from build123d import *

# Parameters (mm, degrees)
ESQUISSE1_R             = 0.65
BOSS_EXTRU_1_DEPTH      = 1
BOSS_EXTRU_2_DEPTH      = 0.6
ESQUISSE4_R             = 0.7
BOSS_EXTRU_3_DEPTH      = 1.8
CHANFREIN1_SIZE         = 0.05
CHANFREIN2_SIZE         = 0.05
ESQUISSE5_R             = 0.575
ENL_V_MAT_EXTRU_1_DEPTH = 2.4
ESQUISSE6_R             = 0.55
ENL_V_MAT_EXTRU_2_DEPTH = 2.4
CHANFREIN3_SIZE         = 0.05
CHANFREIN4_SIZE         = 0.05
CHANFREIN5_SIZE         = 0.01
ESQUISSE7_R             = 0.075
BOSS_EXTRU_4_DEPTH      = 1.5
ECHELLE1_SCALE          = 10


with BuildPart() as part:
    # Esquisse1 → Boss.-Extru.1 (new body)
    with BuildSketch(Plane(origin=(0, 0, 0), x_dir=(0, 0, -1), z_dir=(1, 0, 0))):
        Circle(ESQUISSE1_R)
    extrude(amount=BOSS_EXTRU_1_DEPTH)

    # Esquisse2 → Révolution1 (revolve)
    with BuildSketch(Plane.XY):
        with BuildLine():
            Line((0, 0.65), (0.15, 0.65))
            ThreePointArc((0.15, 0.65), (0.075, 0.725), (0, 0.65))
        make_face()
    revolve(axis=Axis((1, 0, 0), (-1, 0, 0)))

    # Esquisse3 → Boss.-Extru.2 (add)
    with BuildSketch(Plane.ZY):
        Polygon((0.713221279, -0.587067918), (0.86502637, 0.324133787), (0.151805091, 0.911201705), (-0.713221279, 0.587067918), (-0.86502637, -0.324133787), (-0.151805091, -0.911201705), align=None)
    extrude(amount=BOSS_EXTRU_2_DEPTH)

    # Esquisse4 → Boss.-Extru.3 (add)
    with BuildSketch(Plane.ZY.offset(0.6)):
        Circle(ESQUISSE4_R)
    extrude(amount=BOSS_EXTRU_3_DEPTH)

    # Chanfrein1
    chanfrein1_edges = [part.edges().sort_by_distance(p)[0] for p in [
        (-0.6, -0.749134812, 0.280708094),
        (-0.6, -0.131467065, 0.789123825),
        (-0.6, 0.617667746, 0.508415731),
        (-0.6, 0.749134812, -0.280708094),
        (-0.6, 0.131467065, -0.789123825),
        (-0.6, -0.617667746, -0.508415731),
    ]]
    chamfer(chanfrein1_edges, length=CHANFREIN1_SIZE)

    # Chanfrein2
    chanfrein2_edges = [part.edges().sort_by_distance(p)[0] for p in [
        (0, 0.749134812, -0.280708094),
        (0, 0.131467065, -0.789123825),
        (0, -0.617667746, -0.508415731),
        (0, -0.749134812, 0.280708094),
        (0, -0.131467065, 0.789123825),
        (0, 0.617667746, 0.508415731),
    ]]
    chamfer(chanfrein2_edges, length=CHANFREIN2_SIZE)

    # Esquisse5 → Enlèv. mat.-Extru.1 (cut)
    with BuildSketch(Plane.ZY.offset(2.4)):
        Circle(ESQUISSE5_R)
    extrude(amount=-ENL_V_MAT_EXTRU_1_DEPTH, mode=Mode.SUBTRACT)

    # Esquisse6 → Enlèv. mat.-Extru.2 (cut)
    with BuildSketch(Plane(origin=(1, 0, 0), x_dir=(0, 0, -1), z_dir=(1, 0, 0))):
        Circle(ESQUISSE6_R)
    extrude(amount=-ENL_V_MAT_EXTRU_2_DEPTH, mode=Mode.SUBTRACT)

    # Chanfrein3
    chanfrein3_edges = [part.edges().sort_by_distance(p)[0] for p in [
        (1, 0, 0.65),
    ]]
    chamfer(chanfrein3_edges, length=CHANFREIN3_SIZE)

    # Chanfrein4
    chanfrein4_edges = [part.edges().sort_by_distance(p)[0] for p in [
        (-2.4, 0, -0.7),
    ]]
    chamfer(chanfrein4_edges, length=CHANFREIN4_SIZE)

    # Chanfrein5
    chanfrein5_edges = [part.edges().sort_by_distance(p)[0] for p in [
        (-0.6, 0, -0.7),
    ]]
    chamfer(chanfrein5_edges, length=CHANFREIN5_SIZE)

    # Esquisse7 → Boss.-Extru.4 (add)
    with BuildSketch(Plane(origin=(0, 0.617667746, 0.508415731), x_dir=(1, 0, 0), z_dir=(0, 0.772084683, 0.635519663))):
        with Locations((-0.3, 0)):
            Circle(ESQUISSE7_R)
    extrude(amount=-BOSS_EXTRU_4_DEPTH)


with BuildPart() as part_1:
    # Echelle1: scaled about (0, 0, 0)
    add(part.part.scale(ECHELLE1_SCALE))


solid = part_1.part
The listing builds one solid part. Answer for the finished solid, in the listing's coordinates (mm). A direction names the side the tool comes from. Coordinates: 2 decimals unless noted, no trailing zeros. Write each loop counter-clockwise with the first axis right and the second up, starting at its lowest first coordinate (ties: lowest second). Pieces come first, ordered by that corner, then holes. Notation, with made-up numbers: M -23.75,-21 L -3.75,-21 A20 cw -3.75,-10 Z; hole C 87.5,50.25 d3. An arc over 180 degrees is marked long. Use one line per item in the form item = value.
Item 1: Given P1, Ø5, axis at x = 2, y = 1.5, coming from the -Z side; P2, Ø8, axis at x = -20, y = -4.5, coming from the +Z side; P3, Ø3, axis at x = -7, y = -4.5, coming from the -Z side, each flat-ended and moving along its own axis, determine where each tip first touches the part or whether it passes through.
Model answer:
P1 = -7.89
P2 = 6.98
P3 = -7.74
Item 2: Find section C-C, the plane y = 7.75. Give the vertices of the cut face in (x, z), plus the area to 3 significant figures.
Model answer:
outline = M -6,-0.69 L -5.5,-2.12 L -0.5,-2.12 L 0,-0.69 L 0,2.39 L -0.5,3.17 L -5.5,3.17 L -6,2.39 Z
area = 30.6 mm2
Item 3: Find section A-A, the plane x = -4.5. Give the vertices of the cut face in (y, z), plus the area to 3 significant figures.
Model answer:
outline = M -9.11,-1.52 L -3.24,-8.65 L 5.87,-7.13 L 9.11,1.52 L 3.24,8.65 L -5.87,7.13 Z; hole C 0,0 d11.5
area = 118 mm2
Item 4: Find section B-B, the plane z = 0. Give the number of separate pieces and of enclosed holes in the cut face, plus the area to 3 significant figures.
Model answer:
separate_pieces = 3
enclosed_holes = 0
area = 102 mm2
Item 5: The mould has two halves that part along Y. Classify faces 3 (the face through (-0.254, -5.945, -4.977)), 4 (the face through (5.07, -5.37, 1.19)), 5 (the face through (-0.25, 7.28, -2.66)), 6 (the face through (-3.595, -0.228, 0.404)): released by +Y, released by -Y, zero draft, split by the parting line, or undercut.
Model answer:
face_3 = released by -Y
face_4 = undercut
face_5 = released by +Y
face_6 = undercut
Item 6: For faces 1 (the face through (5.44, 1.95, -6.2)), 2 (the face through (-5.746, -5.945, -4.977)), determine the directions among +Z, -Z, +X, -X, +Y, -Y from which every point of the face is accessible in a straight line to the end or side of a thin tool.
Model answer:
face_1 = +X
face_2 = -Z, -X, -Y
Item 7: Find the intervals of material crossed by probe 1 along Z at (x, y) = (-11, 0.25); probe 2 along Y at (x, z) = (-10.25, 0); probe 3 along Z at (x, y) = (-2.5, -3.5), in increasing order.
Model answer:
probe_1 = -7 to -5.74, 5.74 to 7
probe_2 = -7 to -5.75, 5.75 to 7
probe_3 = -8.34 to -4.56, -3.6 to -2.16, 4.56 to 7.53
